from build123d import *

# Parameters (mm, degrees)
F1_DEPTH = 4
F3_DEPTH = 25
F4_D     = 6.8
F4_DEPTH = 15.35
F4_TIP   = 2.0429261047


with BuildPart() as f1:
    # F0 (on Front) → F1 (new body)
    with BuildSketch(Plane.XZ):
        Polygon((0, 55), (0, 0), (35, 0), (35, 20), (15, 55), align=None)
    extrude(amount=F1_DEPTH)

    # F2 (on face) → F3 (cut)
    with BuildSketch(Plane.XZ.offset(4)):
        with BuildLine():
            ThreePointArc((31, 1.25), (32.9445436483, 2.0554563517), (33.75, 4))
            ThreePointArc((33.75, 4), (32.9445436483, 5.9445436483), (31, 6.75))
            ThreePointArc((31, 6.75), (29.910966294, 6.5251743677), (29, 5.8874586088))
            ThreePointArc((29, 5.8874586088), (29.5556310375, 5.0155048006), (29.75, 4))
            ThreePointArc((29.75, 4), (29.5556310375, 2.9844951994), (29, 2.1125413912))
            ThreePointArc((29, 2.1125413912), (29.910966294, 1.4748256323), (31, 1.25))
        make_face()
        with BuildLine():
            ThreePointArc((29, 5.8874586088), (29.910966294, 6.5251743677), (31, 6.75))
            Line((31, 6.75), (27, 6.75))
            ThreePointArc((27, 6.75), (28.089033706, 6.5251743677), (29, 5.8874586088))
        make_face()
        with BuildLine():
            Line((27, 1.25), (31, 1.25))
            ThreePointArc((31, 1.25), (29.910966294, 1.4748256323), (29, 2.1125413912))
            ThreePointArc((29, 2.1125413912), (28.089033706, 1.4748256323), (27, 1.25))
        make_face()
        with BuildLine():
            ThreePointArc((29, 2.1125413912), (28.25, 4), (29, 5.8874586088))
            ThreePointArc((29, 5.8874586088), (28.089033706, 6.5251743677), (27, 6.75))
            ThreePointArc((27, 6.75), (24.25, 4), (27, 1.25))
            ThreePointArc((27, 1.25), (28.089033706, 1.4748256323), (29, 2.1125413912))
        make_face()
        with BuildLine():
            ThreePointArc((16, 1.25), (17.9445436483, 2.0554563517), (18.75, 4))
            ThreePointArc((18.75, 4), (17.9445436483, 5.9445436483), (16, 6.75))
            ThreePointArc((16, 6.75), (14.910966294, 6.5251743677), (14, 5.8874586088))
            ThreePointArc((14, 5.8874586088), (14.5556310375, 5.0155048006), (14.75, 4))
            ThreePointArc((14.75, 4), (14.5556310375, 2.9844951994), (14, 2.1125413912))
            ThreePointArc((14, 2.1125413912), (14.910966294, 1.4748256323), (16, 1.25))
        make_face()
        with BuildLine():
            ThreePointArc((14, 5.8874586088), (14.910966294, 6.5251743677), (16, 6.75))
            Line((16, 6.75), (12, 6.75))
            ThreePointArc((12, 6.75), (13.089033706, 6.5251743677), (14, 5.8874586088))
        make_face()
        with BuildLine():
            Line((12, 1.25), (16, 1.25))
            ThreePointArc((16, 1.25), (14.910966294, 1.4748256323), (14, 2.1125413912))
            ThreePointArc((14, 2.1125413912), (13.089033706, 1.4748256323), (12, 1.25))
        make_face()
        with BuildLine():
            ThreePointArc((14, 2.1125413912), (13.25, 4), (14, 5.8874586088))
            ThreePointArc((14, 5.8874586088), (13.089033706, 6.5251743677), (12, 6.75))
            ThreePointArc((12, 6.75), (9.25, 4), (12, 1.25))
            ThreePointArc((12, 1.25), (13.089033706, 1.4748256323), (14, 2.1125413912))
        make_face()
        with BuildLine():
            ThreePointArc((14.75, 4), (14.5556310375, 5.0155048006), (14, 5.8874586088))
            ThreePointArc((14, 5.8874586088), (13.25, 4), (14, 2.1125413912))
            ThreePointArc((14, 2.1125413912), (14.5556310375, 2.9844951994), (14.75, 4))
        make_face()
        with BuildLine():
            ThreePointArc((29.75, 4), (29.5556310375, 5.0155048006), (29, 5.8874586088))
            ThreePointArc((29, 5.8874586088), (28.25, 4), (29, 2.1125413912))
            ThreePointArc((29, 2.1125413912), (29.5556310375, 2.9844951994), (29.75, 4))
        make_face()
    extrude(amount=-F3_DEPTH, mode=Mode.SUBTRACT)

    # F4
    with Locations(Plane.XZ.offset(4)):
        with Locations((6, 49)):
            Hole(F4_D / 2, depth=F4_DEPTH)
            with Locations((0, 0, -(F4_DEPTH + F4_TIP / 2))):  # 118° drill point
                Cone(0, F4_D / 2, F4_TIP, mode=Mode.SUBTRACT)


solid = f1.part
The listing builds one solid part. Answer for the finished solid, in the listing's coordinates (mm). A direction names the side the tool comes from. Coordinates: 2 decimals unless noted, no trailing zeros. Loops run counter-clockwise (first coordinate to the right, second up) from the corner with the lowest first, then second, coordinate; pieces in that order, holes last. Notation, with made-up numbers: (63.25, -21) -> (96.25, -21) arc R23 cw to (96.25, -13) -> close; hole circle Ø7 at (-38.5, -22.75). An arc over 180 degrees is marked (long way). Write item = value, one per line. Start each with the question number.
1) Given pin 1 Ø1.5 at (y, z) = (-0.5, 33.5) entering from +X; pin 2 Ø1.5 at (x, z) = (13.5, 31) entering from +Y, each flat-ended and moving along its own axis, determine where each tip first touches the part or whether it passes through.
2) A cutting plane is placed at B-B (y = -3.4). Give the vertices of the cut face in (x, z), then the cut area to 3 significant figures.
3) Straight lines are drawn through the part: line 1 (Z direction, x = 6, y = -1); line 2 (X direction, y = -1.1, z = 5.5); line 3 (Z direction, x = 10, y = -3.25). For each, find the intervals that lie inside material, in ascending order. Write a range as from..to.
4) A cutting plane is placed at A-A (x = 6). Give the vertices of the cut face in (y, z), then the cut area to 3 significant figures.
5) The mould has two halves that part along X. Classify faces 3 (the face through (35, -2, 10)), 4 (the face through (24.25, -2.03, 4.06)), 5 (the face through (8, -2, 55)), 6 (the face through (29, -2, 6.75)): released by +X, released by -X, zero draft, split by the parting line, or undercut.
6) A cutting plane is placed at D-D (x = 22). Give the vertices of the cut face in (y, z).
7) A tool of negligible diameter and unlimited length cuts with its end or side. For faces 1 (the face through (25.14, -1.972, 37.255)), 2 (the face through (14, -2, 6.75)), from which of +Z, -Z, +X, -X, +Y, -Y can it reach the whole face along a straight path? Write none if from no direction.
8) A cutting plane is placed at C-C (z = 47.5). Give the vertices of the cut face in (x, y), then the cut area to 3 significant figures.
Responses:
q1.pin_1 = 27.71
q1.pin_2 = 0
q2.outline = (0, 0) -> (35, 0) -> (35, 20) -> (15, 55) -> (0, 55) -> close; hole circle Ø6.8 at (6, 49); hole (12, 1.25) -> (16, 1.25) arc R2.75 ccw to (16, 6.75) -> (12, 6.75) arc R2.75 ccw to start; hole (27, 1.25) -> (31, 1.25) arc R2.75 ccw to (31, 6.75) -> (27, 6.75) arc R2.75 ccw to start
q2.area = 1,450 mm²
q3.line_1 = 0..45.6, 52.4..55
q3.line_2 = 0..9.7, 18.3..24.7, 33.3..35
q3.line_3 = 0..2.11, 5.89..55
q4.outline = (-4, 0) -> (0, 0) -> (0, 45.6) -> (-4, 45.6) -> close; (-4, 52.4) -> (0, 52.4) -> (0, 55) -> (-4, 55) -> close
q4.area = 193 mm²
q5.face_3 = released by +X
q5.face_4 = undercut
q5.face_5 = zero draft
q5.face_6 = undercut
q6.outline = (-4, 0) -> (0, 0) -> (0, 42.75) -> (-4, 42.75) -> close
q7.face_1 = +Z, +X, +Y, -Y
q7.face_2 = +Y, -Y
q8.outline = (0, -4) -> (2.95, -4) -> (2.95, 0) -> (0, 0) -> close; (9.05, -4) -> (19.29, -4) -> (19.29, 0) -> (9.05, 0) -> close
q8.area = 52.7 mm²
